Read the model definition and answer for the solid it produces. Units are mm, in the model's axes. A direction names the side the tool comes from. Round coordinates to 2 decimals unless told otherwise and drop trailing zeros. Order: outer loops, then holes, each group sorted by start corner. A loop starts at its lowest first (then second) coordinate and runs counter-clockwise, first axis right, second up. Notation, with made-up numbers: (-8.75, 89.25) -> (38.25, 89.25) arc R14 ccw to (38.25, 98.25) -> close; hole circle Ø4 at (-12, -24.75). An arc over 180 degrees is marked (long way). Use a Markdown table: item, result. Add a question column.
1. Section A-A, the plane z = -12 is taken. Give the number of separate pieces and of enclosed holes in the cut face, then the cut area to 3 significant figures.
2. Section D-D, the plane y = 6.75 is taken. Give the vertices of the cut face in (x, z).
3. Given pin 1 (6 mm diameter, centred on y = 9.5, z = -20, fed in from +X); pin 2 (12 mm diameter, centred on x = -12, y = 73, fed in from +Z), each flat-ended and moving along its own axis, determine where each tip first touches the part or whether it passes through.
4. Section C-C, the plane y = 66 is taken. Give the vertices of the cut face in (x, z), then the cut area to 3 significant figures.
5. Consider L1, parallel to Z at x = -26.45, y = 75; L2, parallel to Y at x = -26.35, z = -20.75; L3, parallel to X at y = 48.5, z = -6. Determine where each line is inside the solid, lowest interval first. Write a range as [from, to].
6. The mould has two halves that part along X. Classify faces 1 (the face through (5.11, 59.52, -46.06)), 2 (the face through (0, 67, -50)): +X half, -X half, draft (parallel to the pull), parting line (faces both ways), or undercut.
7. Section B-B, the plane x = -9 is taken. Give the vertices of the cut face in (y, z).
8. For faces 3 (the face through (24.25, 25, -26)), 4 (the face through (-24.63, 16.784, -33.134)), 5 (the face through (-25, 22, -10)), 6 (the face through (-4.18, 70.914, -46.056)), determine the directions among +Z, -Z, +X, -X, +Y, -Y from which every point of the face is accessible in a straight line to the end or side of a thin tool.
```python
from build123d import *

# Parameters (mm, degrees)
BOSS_EXTRUDE1_DEPTH = 90
SKETCH2_R           = 10.1
CUT_EXTRUDE1_DEPTH  = 2.8
SKETCH3_R           = 2.5
SKETCH3_R_2         = 1
CUT_EXTRUDE2_DEPTH  = 2.8
SKETCH4_R           = 10.1
CUT_EXTRUDE3_DEPTH  = 2.8
SKETCH5_R           = 2.5
SKETCH5_R_2         = 1
CUT_EXTRUDE4_DEPTH  = 2.8
SKETCH6_R           = 10.025
CUT_EXTRUDE5_DEPTH  = 12.8
CUT_EXTRUDE7_DEPTH  = 62.8
FILLET1_R           = 10
SKETCH9_W           = 1
SKETCH9_H           = 35
CUT_EXTRUDE8_DEPTH  = 50
CUT_EXTRUDE10_DEPTH = 10


with BuildPart() as part:
    # Sketch1 → Boss-Extrude1 (new body)
    with BuildSketch(Plane(origin=(0, 0, 0), x_dir=(1, 0, 0), z_dir=(0, 1, 0))):
        Polygon((-23.25, 0), (-23.25, 42), (23.25, 42), (23.25, 0), (26.25, 0), (26.25, 50), (-27.25, 50), (-27.25, 0), align=None)
    extrude(amount=BOSS_EXTRUDE1_DEPTH)

    # Sketch2 → Cut-Extrude1 (cut)
    with BuildSketch(Plane(origin=(-23.25, 0, 0), x_dir=(0, 0, -1), z_dir=(1, 0, 0))):
        with Locations((12, 78)):
            Circle(SKETCH2_R)
    extrude(amount=-CUT_EXTRUDE1_DEPTH, mode=Mode.SUBTRACT)

    # Sketch3 → Cut-Extrude2 (cut)
    with BuildSketch(Plane(origin=(-26.05, 0, 0), x_dir=(0, 0, -1), z_dir=(1, 0, 0))):
        with Locations((12, 78)):
            Circle(SKETCH3_R)
        with Locations((12, 85)):
            Circle(SKETCH3_R_2)
        with Locations((9, 85)):
            Circle(SKETCH3_R_2)
        with Locations((15, 85)):
            Circle(SKETCH3_R_2)
        with Locations((19, 78)):
            Circle(SKETCH3_R_2)
        with Locations((19, 81)):
            Circle(SKETCH3_R_2)
        with Locations((19, 75)):
            Circle(SKETCH3_R_2)
        with Locations((12, 71)):
            Circle(SKETCH3_R_2)
        with Locations((15, 71)):
            Circle(SKETCH3_R_2)
        with Locations((9, 71)):
            Circle(SKETCH3_R_2)
        with Locations((5, 78)):
            Circle(SKETCH3_R_2)
        with Locations((5, 75)):
            Circle(SKETCH3_R_2)
        with Locations((5, 81)):
            Circle(SKETCH3_R_2)
    extrude(amount=-CUT_EXTRUDE2_DEPTH, mode=Mode.SUBTRACT)

    # Sketch4 → Cut-Extrude3 (cut)
    with BuildSketch(Plane(origin=(-23.25, 0, 0), x_dir=(0, 0, -1), z_dir=(1, 0, 0))):
        with Locations((23.5, 13.75)):
            Circle(SKETCH4_R)
    extrude(amount=-CUT_EXTRUDE3_DEPTH, mode=Mode.SUBTRACT)

    # Sketch5 → Cut-Extrude4 (cut)
    with BuildSketch(Plane(origin=(-26.05, 0, 0), x_dir=(0, 0, -1), z_dir=(1, 0, 0))):
        with Locations((23.75, 13.75)):
            Circle(SKETCH5_R)
        with Locations((23.75, 20.75)):
            Circle(SKETCH5_R_2)
        with Locations((20.75, 20.75)):
            Circle(SKETCH5_R_2)
        with Locations((26.75, 20.75)):
            Circle(SKETCH5_R_2)
        with Locations((30.75, 16.75)):
            Circle(SKETCH5_R_2)
        with Locations((30.75, 13.75)):
            Circle(SKETCH5_R_2)
        with Locations((30.75, 10.75)):
            Circle(SKETCH5_R_2)
        with Locations((26.75, 6.75)):
            Circle(SKETCH5_R_2)
        with Locations((23.75, 6.75)):
            Circle(SKETCH5_R_2)
        with Locations((20.75, 6.75)):
            Circle(SKETCH5_R_2)
        with Locations((16.75, 10.75)):
            Circle(SKETCH5_R_2)
        with Locations((16.75, 13.75)):
            Circle(SKETCH5_R_2)
        with Locations((16.75, 16.75)):
            Circle(SKETCH5_R_2)
    extrude(amount=-CUT_EXTRUDE4_DEPTH, mode=Mode.SUBTRACT)

    # Sketch6 → Cut-Extrude5 (cut)
    with BuildSketch(Plane.ZY.offset(-23.25)):
        with Locations((-12, 78)):
            Circle(SKETCH6_R)
        with Locations((-23.75, 13.75)):
            Circle(SKETCH6_R)
    extrude(amount=-CUT_EXTRUDE5_DEPTH, mode=Mode.SUBTRACT)

    # Sketch8 → Cut-Extrude7 (cut)
    with BuildSketch(Plane.ZY.offset(27.25)):
        with BuildLine():
            Line((0, 60), (-6.83281573, 46.33436854))
            ThreePointArc((-6.83281573, 46.33436854), (-9.197469684, 39.810548291), (-10, 32.917960675))
            Line((-10, 32.917960675), (-10, 0))
            Line((-10, 0), (0, 0))
            Line((0, 0), (0, 60))
        make_face()
        with BuildLine():
            Line((-50, 45), (-49.384007447, 45))
            ThreePointArc((-49.384007447, 45), (-46.548633561, 44.118331571), (-44.713203531, 41.784261971))
            ThreePointArc((-44.713203531, 41.784261971), (-39.074197476, 21.242984276), (-37.5, 0))
            Line((-37.5, 0), (-50, 0))
            Line((-50, 0), (-50, 45))
        make_face()
    extrude(amount=-CUT_EXTRUDE7_DEPTH, mode=Mode.SUBTRACT)

    # Fillet1
    fillet1_edges = [part.edges().sort_by_distance(p)[0] for p in [
        (24.75, 0, -37.5),
        (-25.25, 0, -37.5),
        (-25.25, 0, -10),
        (24.75, 0, -10),
        (-25.25, 60, 0),
        (24.75, 60, 0),
        (24.75, 90, 0),
        (-25.25, 90, 0),
    ]]
    fillet(fillet1_edges, radius=FILLET1_R)

    # Sketch9 → Cut-Extrude8 (cut)
    with BuildSketch(Plane.XY):
        with Locations((23.75, 17.5)):
            Rectangle(SKETCH9_W, SKETCH9_H)
    extrude(amount=-CUT_EXTRUDE8_DEPTH, mode=Mode.SUBTRACT)

    # Sketch10 → Cut-Extrude10 (cut)
    with BuildSketch(Plane(origin=(0, 0, -50), x_dir=(-1, 0, 0), z_dir=(0, 0, -1))):
        with BuildLine():
            ThreePointArc((-5.545477523, 73.609473243), (-2.815070752, 71.565748615), (-0.314206668, 69.246781102))
            Line((-0.314206668, 69.246781102), (-0.718251382, 68.789336849))
            ThreePointArc((-0.718251382, 68.789336849), (-3.14462395, 70.886777127), (-5.763285342, 72.738574113))
            ThreePointArc((-5.763285342, 72.738574113), (-10.24623891, 65.875737216), (-12.109021951, 57.892915514))
            ThreePointArc((-12.109021951, 57.892915514), (-9.506202014, 64.812112187), (-5.398575101, 70.958440796))
            ThreePointArc((-5.398575101, 70.958440796), (-3.57730753, 69.344405913), (-1.663670975, 67.841036595))
            ThreePointArc((-1.663670975, 67.841036595), (-5.130037281, 59.38820373), (-4.32695717, 50.287591599))
            ThreePointArc((-4.32695717, 50.287591599), (-4.15407751, 59.927406093), (0.5, 68.371070782))
            ThreePointArc((0.5, 68.371070782), (5.15407751, 59.927406093), (5.32695717, 50.287591599))
            ThreePointArc((5.32695717, 50.287591599), (6.130037281, 59.38820373), (2.663670975, 67.841036595))
            ThreePointArc((2.663670975, 67.841036595), (4.57730753, 69.344405913), (6.398575101, 70.958440796))
            ThreePointArc((6.398575101, 70.958440796), (10.506202014, 64.812112187), (13.109021951, 57.892915514))
            ThreePointArc((13.109021951, 57.892915514), (11.24623891, 65.875737216), (6.763285342, 72.738574113))
            ThreePointArc((6.763285342, 72.738574113), (4.14462395, 70.886777127), (1.718251382, 68.789336849))
            Line((1.718251382, 68.789336849), (1.314206668, 69.246781102))
            ThreePointArc((1.314206668, 69.246781102), (3.815070752, 71.565748615), (6.545477523, 73.609473243))
            ThreePointArc((6.545477523, 73.609473243), (5.969361402, 80.609191571), (3.438503197, 87.160735145))
            ThreePointArc((3.438503197, 87.160735145), (4.689876448, 80.708142635), (5.106185309, 74.148525875))
            ThreePointArc((5.106185309, 74.148525875), (2.663670975, 72.36347608), (0.5, 70.249047799))
            ThreePointArc((0.5, 70.249047799), (-1.663670975, 72.36347608), (-4.106185309, 74.148525875))
            ThreePointArc((-4.106185309, 74.148525875), (-3.689876448, 80.708142635), (-2.438503197, 87.160735145))
            ThreePointArc((-2.438503197, 87.160735145), (-4.969361402, 80.609191571), (-5.545477523, 73.609473243))
        make_face()
    extrude(amount=-CUT_EXTRUDE10_DEPTH, mode=Mode.SUBTRACT)


solid = part.part
```
Verdict:
| question | item | result |
|---|---|---|
| 1 | separate pieces | 6 |
| 1 | enclosed holes | 0 |
| 1 | area | 443 mm2 |
| 2 | outline | (-27.25, -37.16) -> (-23.25, -37.16) -> (-23.25, -30.78) -> (-26.05, -30.78) -> (-26.05, -27.75) -> (-27.25, -27.75) -> close; (-27.25, -25.75) -> (-26.05, -25.75) -> (-26.05, -24.75) -> (-27.25, -24.75) -> close; (-27.25, -22.75) -> (-26.05, -22.75) -> (-26.05, -21.75) -> (-27.25, -21.75) -> close; (-27.25, -19.75) -> (-26.05, -19.75) -> (-26.05, -16.22) -> (-23.25, -16.22) -> (-23.25, -10.54) -> (-27.25, -10.54) -> close; (24.25, -37.16) -> (26.25, -37.16) -> (26.25, -30.93) -> (24.25, -30.93) -> close; (24.25, -16.57) -> (26.25, -16.57) -> (26.25, -10.54) -> (24.25, -10.54) -> close |
| 3 | pin 1 | stops at x = -26.05 |
| 3 | pin 2 | stops at z = -42 |
| 4 | outline | (-27.25, -50) -> (-11.19, -50) -> (-11.19, -42) -> (-23.25, -42) -> (-23.25, 0) -> (-27.25, 0) -> close; (-9.86, -50) -> (-3.85, -50) -> (-3.85, -42) -> (-9.86, -42) -> close; (-2.38, -50) -> (1.38, -50) -> (1.38, -42) -> (-2.38, -42) -> close; (2.85, -50) -> (8.86, -50) -> (8.86, -42) -> (2.85, -42) -> close; (10.19, -50) -> (26.25, -50) -> (26.25, 0) -> (23.25, 0) -> (23.25, -42) -> (10.19, -42) -> close |
| 4 | area | 677 mm2 |
| 5 | L1 | z = [-50, -20], [-18, -6], [-4, 0] |
| 5 | L2 | y = [0, 5.75], [7.75, 19.75], [21.75, 90] |
| 5 | L3 | x = [-27.25, -23.25], [23.25, 26.25] |
| 6 | face 1 | undercut |
| 6 | face 2 | draft |
| 7 | outline | (33.77, -42) arc R110 cw to (41.78, -44.71) arc R5 cw to (45, -49.38) -> (45, -50) -> (67.43, -50) -> (67.43, -42) -> close; (69.96, -50) -> (90, -50) -> (90, -42) -> (69.96, -42) -> close |
| 8 | face 3 | +Z, -Z, -Y |
| 8 | face 4 | none |
| 8 | face 5 | +Z, +X, -X, -Y |
| 8 | face 6 | +Z, -Z |
